```python
from build123d import *

# Parameters (mm, degrees)
SKETCH1_W            = 160
SKETCH1_H            = 80
SKETCH1_W_2          = 150
SKETCH1_H_2          = 70
BOSS_EXTRUDE1_DEPTH  = 2
CHAMFER1_SIZE        = 3.5
M5_CLEARANCE_HOLE1_D = 5.5


with BuildPart() as part:
    # Sketch1 → Boss-Extrude1 (new body)
    with BuildSketch(Plane.XY):
        Rectangle(SKETCH1_W, SKETCH1_H)
        Rectangle(SKETCH1_W_2, SKETCH1_H_2, mode=Mode.SUBTRACT)
    extrude(amount=BOSS_EXTRUDE1_DEPTH)

    # Chamfer1
    chamfer1_edges = [part.edges().sort_by_distance(p)[0] for p in [
        (-75, 35, 1),
        (-75, -35, 1),
        (75, -35, 1),
        (75, 35, 1),
        (80, -40, 1),
        (-80, -40, 1),
        (-80, 40, 1),
        (80, 40, 1),
    ]]
    chamfer(chamfer1_edges, length=CHAMFER1_SIZE)

    # M5 Clearance Hole1 (through all)
    with Locations(Plane(origin=(0, 0, 0), x_dir=(-1, 0, 0), z_dir=(0, 0, -1))):
        with Locations((0, 0), (-75.75, 35.75), (75.75, -35.75), (75.75, 35.75), (-75.75, -35.75)):
            Hole(M5_CLEARANCE_HOLE1_D / 2)


solid = part.part
```
Can you work these out from the model? Positions are in its coordinate system, mm. A direction names the side the tool comes from. Round coordinates to 2 decimals unless told otherwise and drop trailing zeros. Loops run counter-clockwise (first coordinate to the right, second up) from the corner with the lowest first, then second, coordinate; pieces in that order, holes last. Notation, with made-up numbers: (-31, 7.5) -> (-14, 7.5) arc R15 ccw to (-14, 34.5) -> close; hole circle Ø10 at (-32.75, 66.5). An arc over 180 degrees is marked (long way). One line per item, written item: value. Start each with the question number.
1. If we section it at B-B, the plane x = 14.5: Write out the boundary of the cut face in (y, z).
2. If we mould it in two halves opening along X, with no side actions, what happens to faces 1 (the flat face through (-6, 36, 0)), 2 (the cylindrical face through (-78.497, -35.629, 1.014)), 3 (the flat face through (78.3, -38.2, 1)), 4 (the cylindrical face through (73.003, 35.871, 1.014))? For each: pulls with the +X half, pulls with the -X half, needs draft (parallel to the pull), parting line crosses it, or undercut.
3. If we section it at C-C, the plane z = 0.6: Write out the boundary of the cut face in (x, y).
4. If I drill on probe 1 along Y at (x, z) = (-75.75, 1.2); probe 2 along Y at (x, z) = (25, 1.8); probe 3 along X at (y, z) = (13, 1.05), over which ranges is the centre line in solid material (lowest first)?
5. If we section it at A-A, the plane y = -6.5: Write out the boundary of the cut face in (x, z).
6. For pin 1 (7 mm diameter, centred on x = 75.75, y = -35.75, fed in from +Z), with a flat end and sliding along its axis, tell me the tip position at first contact or that it passes through.
7. For faces 5 (the flat face through (-6, 36, 2)), 6 (the flat face through (73.2, 33.3, 1)), which set-ups out of +Z, -Z, +X, -X, +Y, -Y let a thin tool reach every point of the face, with its end or its side?
Calculated:
1. outline: (-40, 0) -> (-35, 0) -> (-35, 2) -> (-40, 2) -> close; (35, 0) -> (40, 0) -> (40, 2) -> (35, 2) -> close
2. face 1: needs draft
2. face 2: undercut
2. face 3: pulls with the +X half
2. face 4: undercut
3. outline: (-80, -36.5) -> (-76.5, -40) -> (76.5, -40) -> (80, -36.5) -> (80, 36.5) -> (76.5, 40) -> (-76.5, 40) -> (-80, 36.5) -> close; hole circle Ø5.5 at (-75.75, -35.75); hole circle Ø5.5 at (-75.75, 35.75); hole (-75, -31.5) -> (-71.5, -35) -> (71.5, -35) -> (75, -31.5) -> (75, 31.5) -> (71.5, 35) -> (-71.5, 35) -> (-75, 31.5) -> close; hole circle Ø5.5 at (75.75, -35.75); hole circle Ø5.5 at (75.75, 35.75)
4. probe 1: y = -40 to -38.5, -33 to 33, 38.5 to 40
4. probe 2: y = -40 to -35, 35 to 40
4. probe 3: x = -80 to -75, 75 to 80
5. outline: (-80, 0) -> (-75, 0) -> (-75, 2) -> (-80, 2) -> close; (75, 0) -> (80, 0) -> (80, 2) -> (75, 2) -> close
6. pin 1: stops at z = 2
7. face 5: +Z, +X, -X, +Y, -Y
7. face 6: +Z, -Z
